Here's how the part is built. I have some questions about the finished solid (model axes, mm). A direction names the side the tool comes from. Round coordinates to 2 decimals unless told otherwise and drop trailing zeros. Order: outer loops, then holes, each group sorted by start corner. A loop starts at its lowest first (then second) coordinate and runs counter-clockwise, first axis right, second up.
Autodesk Inventor part; units mm, degrees
ref_plane "YZ Plane" through (0, 0, 0) normal (1, 0, 0) x (0, 1, 0)
ref_plane "XZ Plane" through (0, 0, 0) normal (0, 1, 0) x (-1, 0, 0)
ref_plane "XY Plane" through (0, 0, 0) normal (0, 0, 1) x (1, 0, 0)
sketch "Sketch1" plane through (0, 0, 0) normal (0, 0, 1) x (1, 0, 0)
  line L0 (-25, -25) -> (25, -25)
  line L1 (25, -25) -> (25, 25)
  line L2 (25, 25) -> (-25, 25)
  line L3 (-25, 25) -> (-25, -25)
  line L4 (-25, -25) -> (25, 25) construction
  line L5 (25, -25) -> (-25, 25) construction
  line L6 (-15, 15) -> (15, 15)
  line L7 (15, 15) -> (15, -15)
  line L8 (15, -15) -> (-15, -15)
  line L9 (-15, -15) -> (-15, 15)
  circle A0 centre (0, 0) radius 11
  circle A1 centre (0, 0) radius 4.25
  circle A2 centre (-17, 21) radius 2
  circle A3 centre (17, 21) radius 2
  circle A4 centre (-17, -21) radius 2
  circle A5 centre (17, -21) radius 2
  dimension "d0" = 50
  dimension "d1" = 50
  dimension "d2" = 10
  dimension "d3" = 22
  dimension "d4" = 8.5
  dimension "d19" = 4
  dimension "d20" = 4
  dimension "d23" = 34
  dimension "d26" = 42
  dimension "d32" = 8
extrude "Extrusion1" add sketch "Sketch1" along normal blind 10 contours L3 L2 L1 L0 | L6 L7 L8 L9 | A0 | A1 | A2 | A3 | A4 | A5
extrude "Extrusion3" cut sketch "Sketch1" along normal blind 9 contours A0
extrude "Extrusion4" cut sketch "Sketch1" along normal through all contours A2 | A3 | A4 | A5
extrude "Extrusion7" cut sketch "Sketch1" along normal through all contours A1
fillet "Fillet1" radius 6 4 edges at (-25, 25, 5) (-25, -25, 5) (25, 25, 5) (25, -25, 5)
sketch "Sketch4" plane through (0, 0, 10) normal (0, 0, 1) x (1, 0, 0)
  circle A0 centre (0, 0) radius 11
  arc A1 (19, -25) -> (25, -19) centre (19, -19) ccw
  line L0 (25, -19) -> (25, 19)
  arc A2 (25, 19) -> (19, 25) centre (19, 19) ccw
  line L1 (19, 25) -> (-19, 25)
  arc A3 (-19, 25) -> (-25, 19) centre (-19, 19) ccw
  line L2 (-25, 19) -> (-25, -19)
  arc A4 (-25, -19) -> (-19, -25) centre (-19, -19) ccw
  line L3 (-19, -25) -> (19, -25)
  circle A5 centre (17, -21) radius 2
  circle A6 centre (-17, -21) radius 2
  circle A7 centre (17, 21) radius 2
  circle A8 centre (-17, 21) radius 2
  circle A9 centre (17, -21) radius 3.55
  circle A10 centre (-17, -21) radius 2
  circle A11 centre (-17, -21) radius 3.55
  circle A12 centre (-17, 21) radius 3.55
  circle A13 centre (17, 21) radius 3.55
  dimension "d46" = 7.1
extrude "Extrusion9" cut sketch "Sketch4" against normal blind 4 contours A6 | A9 | A11 | A12 | A13
fillet "Fillet3" radius 3.5 8 edges at (-23.2426, -23.2426, 10) (0, -25, 10) (23.2426, -23.2426, 10) (25, 0, 10) (23.2426, 23.2426, 10) (0, 25, 10) (-23.2426, 23.2426, 10) (-25, 0, 10)
sketch "Sketch6" plane through (0, 0, 10) normal (0, 0, 1) x (1, 0, 0)
  point P0 (0, 0)
  point P1 (-5.3246, -13.9891)
  point P2 (-11.8716, -14.0197)
  point P3 (-11.7716, -13.9768)
  point P4 (-11.8836, -14.0009)
hole "Hole1" at (-5.3246, -13.9891, 10) at (-11.8836, -14.0009, 10) direction (0, 0, -1) diameter 1.567 depth 6.3 tip angle 118
equation "\"d23\" = d1 - 2 * d32"
equation "\"d26\" = d0 - 2 * d20"
properties part number "gearbox v2"
1) We'd pull the mould along Y, two halves only. Please class faces 1 (the flat face through (-25, 0, 3)), 2 (the flat face through (0, -5, 9)), 3 (the cylindrical face through (-23.289, -23.196, 3.296)): +Y half, -Y half, draft (parallel to the pull), parting line (faces both ways), or undercut.
2) I need wall thicknesses on line 1 (Y direction, x = 17, z = 1.6); line 2 (X direction, y = -21, z = 7.1); line 3 (Y direction, x = -15.5, z = 4.25). Which ranges of each line are inside material? Lowest first, please.
3) I'm going to push flat-ended pins straight in: pin 1 (3.5 mm diameter, centred on x = -16, y = -20.5, fed in from +Z); pin 2 (2 mm diameter, centred on x = -17.5, y = 21, fed in from +Z); pin 3 (1 mm diameter, centred on y = -6.5, z = 8, fed in from +X). Where does each tip first touch, or does it pass through?
4) For faces 4 (the cylindrical face through (-24, 0.27, 8.95)), 5 (the cylindrical face through (16.54, -17.48, 8.03)), which set-ups out of +Z, -Z, +X, -X, +Y, -Y let a thin tool reach every point of the face, with its end or its side?
5) If we section it at A-A (y = 0): Write out the boundary of the cut face in (x, z), plus the area to 3 significant figures.
6) If we section it at D-D (x = 17): Write out the boundary of the cut face in (y, z), plus the area to 3 significant figures.
7) If we section it at B-B (z = 1.5): Write out the boundary of the cut face in (x, y), plus the area to 3 significant figures.
Solutions:
1. face 1: draft
1. face 2: undercut
1. face 3: -Y half
2. line 1: y = -25 to -23, -19 to 19, 23 to 25
2. line 2: x = -24.6 to -20.55, -13.45 to 13.45, 20.55 to 24.6
2. line 3: y = -25 to -22.32, -19.68 to 19.68, 22.32 to 25
3. pin 1: stops at z = 6
3. pin 2: passes through
3. pin 3: stops at x = 24.85
4. face 4: +Z, -X, +Y, -Y
4. face 5: +Z
5. outline: (-25, 0) - (-11, 0) - (-11, 9) - (-4.25, 9) - (-4.25, 10) - (-21.5, 10) arc R3.5 ccw to (-25, 6.5) - close; (4.25, 9) - (11, 9) - (11, 0) - (25, 0) - (25, 6.5) arc R3.5 ccw to (21.5, 10) - (4.25, 10) - close
5. area: 288 mm2
6. outline: (-25, 0) - (-23, 0) - (-23, 6) - (-24.55, 6) - (-24.55, 8.22) arc R3.5 ccw to (-25, 6.5) - close; (-19, 0) - (19, 0) - (19, 6) - (17.45, 6) - (17.45, 10) - (-17.45, 10) - (-17.45, 6) - (-19, 6) - close; (23, 0) - (25, 0) - (25, 6.5) arc R3.5 ccw to (24.55, 8.22) - (24.55, 6) - (23, 6) - close
6. area: 393 mm2
7. outline: (-25, -19) arc R6 ccw to (-19, -25) - (19, -25) arc R6 ccw to (25, -19) - (25, 19) arc R6 ccw to (19, 25) - (-19, 25) arc R6 ccw to (-25, 19) - close; hole circle Ø4 at (-17, -21); hole circle Ø4 at (-17, 21); hole circle Ø22 at (0, 0); hole circle Ø4 at (17, -21); hole circle Ø4 at (17, 21)
7. area: 2,040 mm2
